```python
from build123d import *

# Parameters (mm, degrees)
SKETCH1_W           = 15
SKETCH1_H           = 8
SKETCH1_R           = 2.5
BOSS_EXTRUDE1_DEPTH = 6
FILLET1_R           = 4
SKETCH2_R           = 4
BOSS_EXTRUDE2_DEPTH = 5
SKETCH4_R           = 2.5
CUT_EXTRUDE1_DEPTH  = 25


with BuildPart() as part:
    # Sketch1 → Boss-Extrude1 (new body)
    with BuildSketch(Plane(origin=(0, 0, 0), x_dir=(1, 0, 0), z_dir=(0, 1, 0))):
        Rectangle(SKETCH1_W, SKETCH1_H)
        with Locations(Location((-3.5, 0, 0), (0, 0, 270))):
            Circle(SKETCH1_R, mode=Mode.SUBTRACT)
        with Locations(Location((3.5, 0, 0), (0, 0, 270))):
            Circle(SKETCH1_R, mode=Mode.SUBTRACT)
    extrude(amount=BOSS_EXTRUDE1_DEPTH)

    # Fillet1
    fillet1_edges = [part.edges().sort_by_distance(p)[0] for p in [
        (-7.5, 3, -4),
        (7.5, 3, -4),
        (7.5, 3, 4),
        (-7.5, 3, 4),
    ]]
    fillet(fillet1_edges, radius=FILLET1_R - 0.0001)  # a hair under: the kernel refuses the full size

    # Sketch2 → Boss-Extrude2 (add)
    with BuildSketch(Plane(origin=(0, 6, 0), x_dir=(1, 0, 0), z_dir=(0, 1, 0))):
        with Locations(Location((3.5, 0, 0), (0, 0, 270))):
            Circle(SKETCH2_R)
    extrude(amount=BOSS_EXTRUDE2_DEPTH)

    # Sketch4 → Cut-Extrude1 (cut)
    with BuildSketch(Plane.XZ.offset(-6)):
        with Locations(Location((3.5, 0, 0), (0, 0, 90))):
            Circle(SKETCH4_R)
    extrude(amount=-CUT_EXTRUDE1_DEPTH, mode=Mode.SUBTRACT)


solid = part.part
```
Verification items for the finished model (mm, model axes). Round coordinates to 2 decimals unless told otherwise and drop trailing zeros. Write each loop counter-clockwise with the first axis right and the second up, starting at its lowest first coordinate (ties: lowest second). Pieces come first, ordered by that corner, then holes. Notation, with made-up numbers: (-35.75, -18.5) -> (-24.75, -18.5) arc R19 cw to (-24.75, 17.5) -> close; hole circle Ø2 at (-33, 42.25). An arc over 180 degrees is marked (long way). Write each question's results on one line, items separated by ' | '. Start each with the question number.
1. Cross-section at C-C (x = -4.5). Enter the section's corners in (y, z), then the cut area to 3 significant figures.
2. Draft check along X on faces 1 (the cylindrical face through (6.297, 3.042, 2.859)), 2 (the cylindrical face through (-1.39, 2.96, 1.34)), 3 (the cylindrical face through (-0.405, 8.465, -0.867)), 4 (the cylindrical face through (1.39, 5.42, 1.34)). Enter one of: +X half, -X half, draft (parallel to the pull), parting line (faces both ways), or undercut.
3. Material ranges on probe 1 along X at (y, z) = (4.75, 0); probe 2 along Z at (x, y) = (3.5, 7.5); probe 3 along X at (y, z) = (6.5, 0), recorded low to high. Write a range as from..to.
4. Cross-section at B-B (z = -0.5). Enter the section's corners in (x, y), then the cut area to 3 significant figures.
5. Cross-section at D-D (y = 9.25). Enter the section's corners in (x, z).
6. Cross-section at A-A (y = 4). Count the separate pieces of the cut face and the enclosed holes in it, then the cut area to 3 significant figures.
7. Depth check by flat-ended pin: P1, Ø2, axis at x = -3, z = 1.5, coming from the +Y side; P2, Ø1, axis at y = 3, z = -1, coming from the +X side; P3, Ø2, axis at x = 0.5, y = 8, coming from the -Z side. Enter the tip coordinate at first touch or a pass-through.
Solutions:
1) outline: (0, -3.87) -> (6, -3.87) -> (6, -2.29) -> (0, -2.29) -> close; (0, 2.29) -> (6, 2.29) -> (6, 3.87) -> (0, 3.87) -> close | area: 19.0 mm2
2) face 1: +X half | face 2: undercut | face 3: parting line | face 4: undercut
3) probe 1: x = -7.5..-6, -1..1, 6..7.5 | probe 2: z = -4..-2.5, 2.5..4 | probe 3: x = -0.5..1, 6..7.5
4) outline: (-7.47, 0) -> (-5.95, 0) -> (-5.95, 6) -> (-7.47, 6) -> close; (-1.05, 0) -> (1.05, 0) -> (1.05, 11) -> (-0.47, 11) -> (-0.47, 6) -> (-1.05, 6) -> close; (5.95, 0) -> (7.47, 0) -> (7.47, 11) -> (5.95, 11) -> close | area: 46.0 mm2
5) outline: circle Ø8 at (3.5, 0); hole circle Ø5 at (3.5, 0)
6) separate pieces: 1 | enclosed holes: 2 | area: 67.0 mm2
7) P1: stops at y = 6 | P2: stops at x = 7.47 | P3: stops at z = -3.46
